Input: part model. Units: mm. Frame: model coordinates. Give positions to 0.01 mm unless a question says otherwise; leave off trailing zeros. Write each loop counter-clockwise with the first axis right and the second up, starting at its lowest first coordinate (ties: lowest second). Pieces come first, ordered by that corner, then holes. Notation, with made-up numbers: (76, -32) - (130, -32) arc R29 cw to (130, 7) - close; hole circle Ø9 at (-25, 12.5). An arc over 180 degrees is marked (long way). Answer as CSV lines item,"result".
```python
from build123d import *

# Parameters (mm, degrees)
ESQUISSE1_R               = 1.5
T_LE_DE_BASE_PLI_E1_DEPTH = 1


# Sheet-metal steps are written as plain solids
with BuildPart() as part:
    # Esquisse1 → Tôle de base pliée1 (new body)
    with BuildSketch(Plane.XY):
        with BuildLine():
            Line((-58.469338958, -21.747952398), (-53.848876988, 15.970095876))
            ThreePointArc((-53.848876988, 15.970095876), (-49.26123741, 19.438010656), (-45.943968874, 14.740287881))
            ThreePointArc((-45.943968874, 14.740287881), (-42.861840407, 3.075501185), (-31.856499609, -1.869115936))
            ThreePointArc((-31.856499609, -1.869115936), (-27.76403967, -5.778781082), (-31.673704815, -9.871241021))
            ThreePointArc((-31.673704815, -9.871241021), (-31.985478135, -9.876154218), (-32.297289768, -9.876651277))
            ThreePointArc((-32.297289768, -9.876651277), (-43.713897158, -13.595668804), (-50.642240989, -23.40220068))
            ThreePointArc((-50.642240989, -23.40220068), (-55.314375936, -26.164336213), (-58.469338958, -21.747952398))
        make_face()
        with Locations((-54.484155586, -22.236137473)):
            Circle(ESQUISSE1_R, mode=Mode.SUBTRACT)
        with Locations((-31.765102212, -5.870178479)):
            Circle(ESQUISSE1_R, mode=Mode.SUBTRACT)
        with Locations((-49.876465203, 15.483475321)):
            Circle(ESQUISSE1_R, mode=Mode.SUBTRACT)
    extrude(amount=T_LE_DE_BASE_PLI_E1_DEPTH)


solid = part.part
```
Item 1: Cut plane B-B on z = 0.4. Return the cut outline in (x, y).
The answers:
outline,"(-58.47, -21.75) arc R4.01 ccw to (-50.64, -23.4) arc R19.06 cw to (-32.3, -9.88) arc R22.02 ccw to (-31.67, -9.87) arc R4 ccw to (-31.86, -1.87) arc R14.01 cw to (-45.94, 14.74) arc R4 ccw (long way) to (-53.85, 15.97) - close; hole circle Ø3 at (-54.48, -22.24); hole circle Ø3 at (-49.88, 15.48); hole circle Ø3 at (-31.77, -5.87)"
Item 2: Mould query, pull axis X, two halves, no side actions, for faces 1 (the face through (-48.446, 15.934, 0.493)), 2 (the face through (-46, -3, 1)), 3 (the face through (-56.19, -3.15, 0.49)), 4 (the face through (-55.23, -26.18, 0.49)). Classes: +X half, -X half, draft (parallel to the pull), parting line (faces both ways), or undercut.
The answers:
face 1,"undercut"
face 2,"draft"
face 3,"-X half"
face 4,"parting line"
Item 3: Cut plane A-A on x = -31. Return the cut outline in (y, z), plus the area to 3 significant figures.
The answers:
outline,"(-9.8, 0) - (-7.16, 0) - (-7.16, 1) - (-9.8, 1) - close; (-4.58, 0) - (-1.94, 0) - (-1.94, 1) - (-4.58, 1) - close"
area,"5.28 mm²"
Item 4: Contact query for a flat-ended pin moving along its axis: pin 1 (2.5 mm diameter, centred on x = -31.77, y = -5.87, fed in from +Z). Output: stop coordinate, or through.
The answers:
pin 1,"through"
Item 5: Ray query, line 1 (X direction, y = -4.5, z = 0.25); line 2 (Y direction, x = -48.5, z = 0.1); line 3 (Y direction, x = -31.5, z = 0.2). Return the intervals inside material, ascending. Write a range as from..to.
The answers:
line 1,"-56.36..-32.38, -31.15..-28"
line 2,"-18.73..14.89, 16.08..19.24"
line 3,"-9.86..-7.35, -4.39..-1.88"
Item 6: Cut plane D-D on y = 2.5. Return the cut outline in (x, z), plus the area to 3 significant figures.
The answers:
outline,"(-55.5, 0) - (-42.35, 0) - (-42.35, 1) - (-55.5, 1) - close"
area,"13.2 mm²"
Item 7: Cut plane C-C on x = -49. Return the cut outline in (y, z).
The answers:
outline,"(-19.56, 0) - (14.27, 0) - (14.27, 1) - (-19.56, 1) - close; (16.7, 0) - (19.39, 0) - (19.39, 1) - (16.7, 1) - close"
